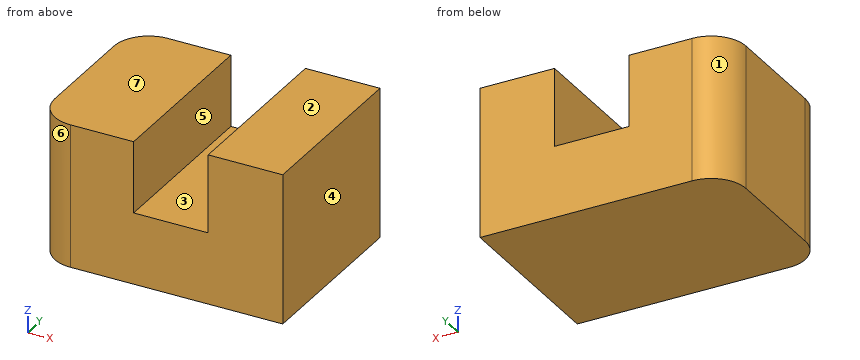
```python
from build123d import *

# Parameters (mm, degrees)
F1_DEPTH = 73.06463
F2_W     = 90.6488774794
F2_H     = 36.532315
F3_DEPTH = 76.2
F4_W     = 38.1
F4_H     = 90.6488774794
F5_DEPTH = 40


with BuildPart() as f1:
    # F0 (on Top) → F1 (new body)
    with BuildSketch(Plane.XY):
        with BuildLine():
            Line((-68.4786736965, 31.1171887892), (-100.6505399656, 31.1171887892))
            ThreePointArc((-100.6505399656, 31.1171887892), (-113.2228985351, 25.9095473587), (-118.4305399656, 13.3371887892))
            Line((-118.4305399656, 13.3371887892), (-118.4305399656, -41.7516886902))
            ThreePointArc((-118.4305399656, -41.7516886902), (-113.2228985351, -54.3240472597), (-100.6505399656, -59.5316886902))
            Line((-100.6505399656, -59.5316886902), (-68.4786736965, -59.5316886902))
            Line((-68.4786736965, -59.5316886902), (-68.4786736965, 31.1171887892))
        make_face()
    extrude(amount=F1_DEPTH)

    # F2 (on face) → F3 (join)
    with BuildSketch(Plane.YZ.offset(-68.4786736965)):
        with Locations((-14.2072499505, 18.2661575)):
            Rectangle(F2_W, F2_H)
    extrude(amount=F3_DEPTH)

    # F4 (on face) → F5 (join)
    with BuildSketch(Plane.XY.offset(36.532315)):
        with Locations((-11.3286736965, -14.2072499505)):
            Rectangle(F4_W, F4_H)
    extrude(amount=F5_DEPTH)


solid = f1.part
```
CAD build for the part. Positions are in the model's coordinates, mm. Face numbers are marked on the shaded views. A direction names the side the tool comes from. Coordinates: 2 decimals unless noted, no trailing zeros. Order: outer loops, then holes, each group sorted by start corner. A loop starts at its lowest first (then second) coordinate and runs counter-clockwise, first axis right, second up. Notation, with made-up numbers: (42.5, -27) - (81.5, -27) arc R7 cw to (81.5, -22) - close; hole circle Ø4 at (22, 66.25). An arc over 180 degrees is marked (long way). Use a Markdown table: item, result. Add a question column.
(1) Drill centre lines: line 1 along X through (y, z) = (-0.5, 67); line 2 along Z through (x, y) = (-86, -38); line 3 along Z through (x, y) = (-63.5, -21). Where is each one in solid material? Low to high. Write a range as [from, to].
(2) Which spindle directions (+Z, -Z, +X, -X, +Y, -Y) get a long thin tool onto all of the face, cutting with end or side? Do the marked faces 5, 6 and 7. Say none if no direction does.
(3) Pull direction X, two halves, no side cores. Call the marked faces 1, 2, 3 and 4: +X half, -X half, draft (parallel to the pull), parting line (faces both ways), or undercut.
(4) Saw through at C-C (x = -58). Give the cut face in (y, z), then the cut area to 3 significant figures.
(5) Flat gauge pins, fed straight in: pin 1 (1.5 mm diameter, centred on x = -92.5, y = -11.5, fed in from -Z); pin 2 (4 mm diameter, centred on x = -55, y = -8, fed in from +Z); pin 3 (15 mm diameter, centred on x = -92, y = 7, fed in from +Z). Where does each tip first touch, or does it go through?
(6) Saw through at B-B (y = -20). Give the cut face in (x, z).
(7) Saw through at D-D (y = 17). Give the cut face in (x, z).
(8) Saw through at A-A (z = 64.5). Give the cut face in (x, y).
Solved:
| question | item | result |
|---|---|---|
| 1 | line 1 | x = [-118.43, -68.48], [-30.38, 7.72] |
| 1 | line 2 | z = [0, 73.06] |
| 1 | line 3 | z = [0, 36.53] |
| 2 | face 5 | +Z, +Y, -Y |
| 2 | face 6 | +Z, -Z, -X, -Y |
| 2 | face 7 | +Z, -X, +Y, -Y |
| 3 | face 1 | -X half |
| 3 | face 2 | draft |
| 3 | face 3 | undercut |
| 3 | face 4 | +X half |
| 4 | outline | (-59.53, 0) - (31.12, 0) - (31.12, 36.53) - (-59.53, 36.53) - close |
| 4 | area | 3,310 mm² |
| 5 | pin 1 | stops at z = 0 |
| 5 | pin 2 | stops at z = 36.53 |
| 5 | pin 3 | stops at z = 73.06 |
| 6 | outline | (-118.43, 0) - (7.72, 0) - (7.72, 76.53) - (-30.38, 76.53) - (-30.38, 36.53) - (-68.48, 36.53) - (-68.48, 73.06) - (-118.43, 73.06) - close |
| 7 | outline | (-118.05, 0) - (7.72, 0) - (7.72, 76.53) - (-30.38, 76.53) - (-30.38, 36.53) - (-68.48, 36.53) - (-68.48, 73.06) - (-118.05, 73.06) - close |
| 8 | outline | (-118.43, -41.75) arc R17.78 ccw to (-100.65, -59.53) - (-68.48, -59.53) - (-68.48, 31.12) - (-100.65, 31.12) arc R17.78 ccw to (-118.43, 13.34) - close; (-30.38, -59.53) - (7.72, -59.53) - (7.72, 31.12) - (-30.38, 31.12) - close |
